The figure shows three views and two pictorial views of one solid part (mm, origin at its lowest corner). Answer the questions. Give positions to 0.01 mm unless a question says otherwise; leave off trailing zeros. Order: outer loops, then holes, each group sorted by start corner. A loop starts at its lowest first (then second) coordinate and runs counter-clockwise, first axis right, second up. Notation, with made-up numbers: (88.5, 87) - (140.5, 87) arc R29 ccw to (140.5, 121) - close; hole circle Ø7 at (-4.5, 64). An arc over 180 degrees is marked (long way). Answer as a JSON object with one key per item and string values. Group by question number.
Q1. A cutting plane is placed at C-C, the plane x = 12.7. Give the vertices of the cut face in (y, z) (1 decimal), and give its area (3 significant figures).
Q2. Consider line 1 (Y direction, x = 12.7, z = 2.75); line 2 (Y direction, x = 26.5, z = 8) (1 decimal); line 3 (Y direction, x = 38.1, z = 3.75). Determine where each line is inside the solid, lowest interval first.
Q3. A cutting plane is placed at B-B, the plane x = 38.1. Give the vertices of the cut face in (y, z) (1 decimal), and give its area (3 significant figures).
Q4. A cutting plane is placed at A-A, the plane y = 25.4. Give the vertices of the cut face in (x, z) (1 decimal), and give its area (3 significant figures).
Q5. A cutting plane is placed at D-D, the plane y = 164. Give the vertices of the cut face in (x, z) (1 decimal), and give its area (3 significant figures).
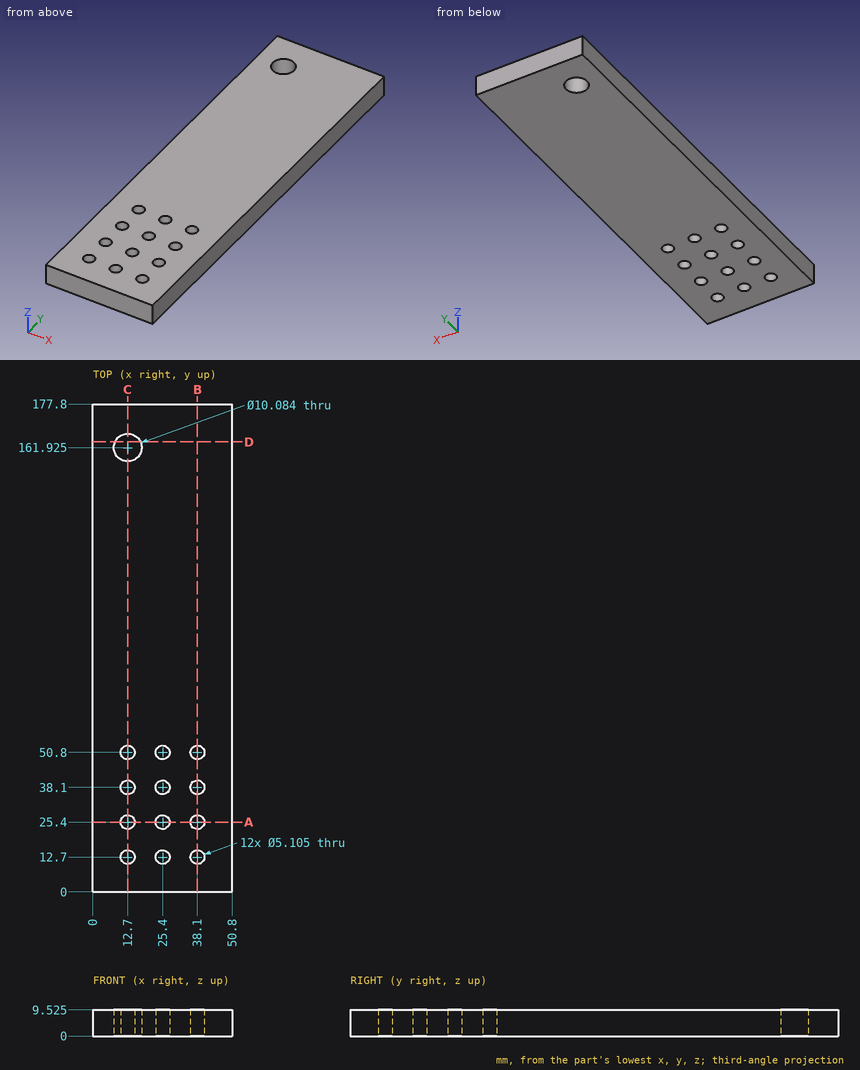
Reply:
{
 "1": {"outline": "(0, 0) - (10.1, 0) - (10.1, 9.5) - (0, 9.5) - close; (15.3, 0) - (22.8, 0) - (22.8, 9.5) - (15.3, 9.5) - close; (28, 0) - (35.5, 0) - (35.5, 9.5) - (28, 9.5) - close; (40.7, 0) - (48.2, 0) - (48.2, 9.5) - (40.7, 9.5) - close; (53.4, 0) - (156.9, 0) - (156.9, 9.5) - (53.4, 9.5) - close; (167, 0) - (177.8, 0) - (177.8, 9.5) - (167, 9.5) - close", "area": "1,400 mm^2"},
 "2": {"line 1": "y = 0 to 10.15, 15.25 to 22.85, 27.95 to 35.55, 40.65 to 48.25, 53.35 to 156.88, 166.97 to 177.8", "line 2": "y = 0 to 10.4, 15 to 23.1, 27.7 to 35.8, 40.4 to 48.5, 53.1 to 177.8", "line 3": "y = 0 to 10.15, 15.25 to 22.85, 27.95 to 35.55, 40.65 to 48.25, 53.35 to 177.8"},
 "3": {"outline": "(0, 0) - (10.1, 0) - (10.1, 9.5) - (0, 9.5) - close; (15.3, 0) - (22.8, 0) - (22.8, 9.5) - (15.3, 9.5) - close; (28, 0) - (35.5, 0) - (35.5, 9.5) - (28, 9.5) - close; (40.7, 0) - (48.2, 0) - (48.2, 9.5) - (40.7, 9.5) - close; (53.4, 0) - (177.8, 0) - (177.8, 9.5) - (53.4, 9.5) - close", "area": "1,500 mm^2"},
 "4": {"outline": "(0, 0) - (10.1, 0) - (10.1, 9.5) - (0, 9.5) - close; (15.3, 0) - (22.8, 0) - (22.8, 9.5) - (15.3, 9.5) - close; (28, 0) - (35.5, 0) - (35.5, 9.5) - (28, 9.5) - close; (40.7, 0) - (50.8, 0) - (50.8, 9.5) - (40.7, 9.5) - close", "area": "338 mm^2"},
 "5": {"outline": "(0, 0) - (8.1, 0) - (8.1, 9.5) - (0, 9.5) - close; (17.3, 0) - (50.8, 0) - (50.8, 9.5) - (17.3, 9.5) - close", "area": "396 mm^2"}
}
